CAD build for the part. Positions are in the model's coordinates, mm. A direction names the side the tool comes from. Round coordinates to 2 decimals unless told otherwise and drop trailing zeros. Order: outer loops, then holes, each group sorted by start corner. A loop starts at its lowest first (then second) coordinate and runs counter-clockwise, first axis right, second up. Notation, with made-up numbers: (-13.75, 76.25) -> (12.25, 76.25) arc R15 cw to (12.25, 94.25) -> close; hole circle Ø1 at (34.5, -17). An arc over 180 degrees is marked (long way). Return JSON: item names as keys, results as strings. Group by question number.
Q1. Probe line 1 along X through (y, z) = (2.25, 21.75); line 2 along Z through (x, y) = (49.5, 21.5); line 3 along Y through (x, z) = (42.5, 8.5). List the from-to ranges inside material, lowest first.
Q2. Cut at D-D (x = 37). Write the cut outline in (y, z), then the cut area to 3 significant figures.
Q3. Which spindle directions (+Z, -Z, +X, -X, +Y, -Y) get a long thin tool onto all of the face, cutting with end or side? Do faces 5 (the flat face through (44, 12.725, 7)), 6 (the flat face through (37.6, 25.4, 12.5)), 7 (the flat face through (50.825, 10, 15)), 8 (the flat face through (35, 15, 13.096)), 9 (the flat face through (63, 0, 13)). Say none if no direction does.
Q4. Cut at C-C (y = 16.5). Write the cut outline in (x, z).
Q5. Cut at B-B (y = 2). Write the cut outline in (x, z), then the cut area to 3 significant figures.
Q6. Flat gauge pins, fed straight in: pin 1 (6.5 mm diameter, centred on x = 42, z = 7.5, fed in from -Y); pin 2 (7.5 mm diameter, centred on x = 42, y = 17.5, fed in from +Z). Where does each tip first touch, or does it go through?
Q7. Cut at A-A (z = 14.25). Write the cut outline in (x, y).
Q8. Mould opens along X. For faces 1 (the flat face through (76.2, 13, 13)), 2 (the flat face through (38, 13, 0)), 3 (the flat face through (0, 13, 13)), 4 (the flat face through (25.375, 13, 19)) say: +X half, -X half, draft (parallel to the pull), parting line (faces both ways), or undercut.
from build123d import *

# Parameters (mm, degrees)
F0_W     = 76.2
F0_H     = 25.4
F1_DEPTH = 25.4
F2_W     = 25.4508
F2_H     = 12.7254
F3_DEPTH = 25.4
F4_W     = 12.7254
F4_H     = 12.7254
F5_DEPTH = 25.4


with BuildPart() as f1:
    # F0 (on Top) → F1 (new body)
    with BuildSketch(Plane.XY):
        with Locations((38.1, 12.7)):
            Rectangle(F0_W, F0_H)
    extrude(amount=F1_DEPTH)

    # F2 (on Front) → F3 (cut)
    with BuildSketch(Plane.XZ):
        with Locations((38.1, 19.458432)):
            Rectangle(F2_W, F2_H)
    extrude(amount=-F3_DEPTH, mode=Mode.SUBTRACT)

    # F4 (on face) → F5 (cut)
    with BuildSketch(Plane.XY.offset(13.095732)):
        with Locations((44.4627, 6.3627)):
            Rectangle(F4_W, F4_H)
    extrude(amount=-F5_DEPTH, mode=Mode.SUBTRACT)


solid = f1.part
Solution:
{
 "1": {"line 1": "x = 0 to 25.37, 50.83 to 76.2", "line 2": "z = 0 to 13.1", "line 3": "y = 12.73 to 25.4"},
 "2": {"outline": "(0, 0) -> (25.4, 0) -> (25.4, 13.1) -> (0, 13.1) -> close", "area": "333 mm²"},
 "3": {"face 5": "+Z, -Z, -Y", "face 6": "+Z, -Z, +X, -X, +Y", "face 7": "+Z, -Y", "face 8": "+Z, +Y, -Y", "face 9": "+Z, -Z, +X, -X, -Y"},
 "4": {"outline": "(0, 0) -> (76.2, 0) -> (76.2, 25.4) -> (50.83, 25.4) -> (50.83, 13.1) -> (25.37, 13.1) -> (25.37, 25.4) -> (0, 25.4) -> close"},
 "5": {"outline": "(0, 0) -> (38.1, 0) -> (38.1, 13.1) -> (25.37, 13.1) -> (25.37, 25.4) -> (0, 25.4) -> close; (50.83, 0) -> (76.2, 0) -> (76.2, 25.4) -> (50.83, 25.4) -> close", "area": "1,460 mm²"},
 "6": {"pin 1": "stops at y = 12.73", "pin 2": "stops at z = 13.1"},
 "7": {"outline": "(0, 0) -> (25.37, 0) -> (25.37, 25.4) -> (0, 25.4) -> close; (50.83, 0) -> (76.2, 0) -> (76.2, 25.4) -> (50.83, 25.4) -> close"},
 "8": {"face 1": "+X half", "face 2": "draft", "face 3": "-X half", "face 4": "undercut"}
}
